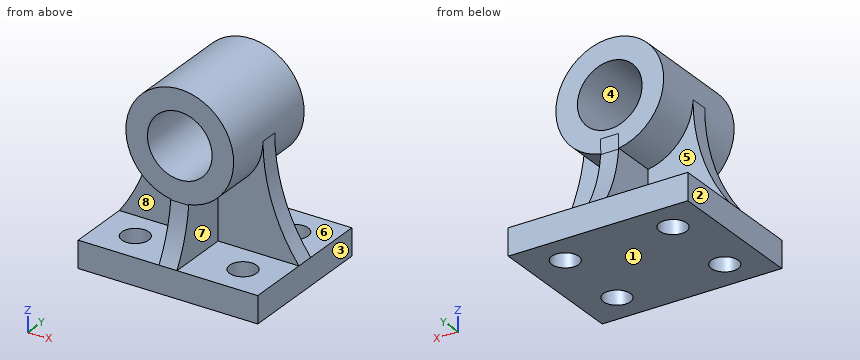
from build123d import *

# Parameters (mm, degrees)
F0_W     = 100
F0_H     = 15
F1_DEPTH = 40
F0_R     = 18
F2_DEPTH = 30
F3_DEPTH = 5
F6_DEPTH = 10
F7_R     = 7.5
F8_DEPTH = 15


with BuildPart() as f1:
    # F0 (on Front) → F1 (new body, symmetric)
    with BuildSketch(Plane.XZ):
        with Locations((50, 7.5)):
            Rectangle(F0_W, F0_H)
    extrude(amount=F1_DEPTH, both=True)



with BuildPart() as f2:
    # F0 (on Front) → F2 (new body, symmetric)
    with BuildSketch(Plane.XZ):
        with BuildLine():
            ThreePointArc((80, 75), (50, 105), (20, 75))
            ThreePointArc((20, 75), (50, 45), (80, 75))
        make_face()
        with Locations((50, 75)):
            Circle(F0_R, mode=Mode.SUBTRACT)
    extrude(amount=F2_DEPTH, both=True)


with BuildPart() as f1_1:
    add(f1.part)

    add(f2.part)  # F3 merges F2
    # F0 (on Front) → F3 (join, symmetric)
    with BuildSketch(Plane.XZ):
        with BuildLine():
            ThreePointArc((20, 75), (14.86833, 43.377223), (0, 15))
            Line((0, 15), (100, 15))
            ThreePointArc((100, 15), (85.13167, 43.377223), (80, 75))
            ThreePointArc((80, 75), (50, 45), (20, 75))
        make_face()
    extrude(amount=F3_DEPTH, both=True)

    # F5 (on offset) → F6 (join)
    with BuildSketch(Plane.YZ.offset(45)):
        with BuildLine():
            ThreePointArc((40, 15), (33.400891, 29.466964), (30, 45))
            Line((30, 45), (30.077839, 53.216796))
            Line((30.077839, 53.216796), (-30, 53.216796))
            Line((-30, 53.216796), (-30, 45))
            ThreePointArc((-30, 45), (-33.400891, 29.466964), (-40, 15))
            Line((-40, 15), (-5, 15))
            Line((-5, 15), (5, 15))
            Line((5, 15), (40, 15))
        make_face()
    extrude(amount=F6_DEPTH)

    # F7 (on face) → F8 (cut, through all)
    with BuildSketch(Plane(origin=(0, 0, 0), x_dir=(1, 0, 0), z_dir=(0, 0, -1))):
        with Locations((80, -22)):
            Circle(F7_R)
        with Locations((20, -22)):
            Circle(F7_R)
        with Locations((80, 22)):
            Circle(F7_R)
        with Locations((20, 22)):
            Circle(F7_R)
    extrude(amount=-F8_DEPTH, mode=Mode.SUBTRACT)


solid = f1_1.part
Work out the finished part from the listing and answer in its coordinate system (mm). Face numbers are marked on the shaded views. A direction names the side the tool comes from. Coordinates: 2 decimals unless noted, no trailing zeros. Loops run counter-clockwise (first coordinate to the right, second up) from the corner with the lowest first, then second, coordinate; pieces in that order, holes last. Notation, with made-up numbers: M -6,8 L 14,8 A10 ccw 14,27 Z; hole C -18.75,83.25 d5. An arc over 180 degrees is marked long. Answer in a Markdown table with one row per item. Add a question column.
1. Find section D-D, the plane z = 87. Write down the section's boundary in (x, y).
2. Find section B-B, the plane x = 50. Write down the section's boundary in (y, z).
3. Flat-ended cylindrical pins translate along their axes: P1, Ø22.5, axis at x = 27.5, z = 59, coming from the -Y side; P2, Ø3, axis at y = -6, z = 56.5, coming from the +X side; P3, Ø9, axis at x = 80, y = -22, coming from the +Z side. Find the tip coordinate at first contact, or state that the pin passes through.
4. A tool of negligible diameter and unlimited length cuts with its end or side. For the marked faces 5, 6, 7 and 8, from which of +Z, -Z, +X, -X, +Y, -Y can it reach the whole face along a straight path? Write none if from no direction.
5. The mould has two halves that part along X. Classify the marked faces 1, 2, 3 and 4: pulls with the +X half, pulls with the -X half, needs draft (parallel to the pull), parting line crosses it, or undercut.
6. Find section A-A, the plane y = 22. Write down the section's boundary in (x, z), then the cut area to 3 significant figures.
7. Find section C-C, the plane y = -6.5. Write down the section's boundary in (x, z).
8. Consider L1, parallel to X at y = -22, z = 6; L2, parallel to Y at x = 20, z = 11; L3, parallel to Z at x = 56.5, y = -22.5. Determine where each line is inside the solid, lowest interval first.
Reported:
| question | item | result |
|---|---|---|
| 1 | outline | M 22.5,-30 L 36.58,-30 L 36.58,30 L 22.5,30 Z; M 63.42,-30 L 77.5,-30 L 77.5,30 L 63.42,30 Z |
| 2 | outline | M -40,0 L 40,0 L 40,15 A75 cw 30,45 L 30.08,53.22 L 30,53.22 L 30,57 L -30,57 L -30,45 A75 cw -40,15 Z; M -30,93 L 30,93 L 30,105 L -30,105 Z |
| 3 | P1 | stops at y = -30 |
| 3 | P2 | stops at x = 81.94 |
| 3 | P3 | stops at z = 90.8 |
| 4 | face 5 | -X, +Y |
| 4 | face 6 | +X, +Y |
| 4 | face 7 | +X, -Y |
| 4 | face 8 | -X, -Y |
| 5 | face 1 | needs draft |
| 5 | face 2 | pulls with the -X half |
| 5 | face 3 | pulls with the +X half |
| 5 | face 4 | undercut |
| 6 | outline | M 0,0 L 12.5,0 L 12.5,15 L 0,15 Z; M 27.5,0 L 72.5,0 L 72.5,15 L 55,15 L 55,45.42 A30 ccw long 45,45.42 L 45,15 L 27.5,15 Z; M 87.5,0 L 100,0 L 100,15 L 87.5,15 Z; hole C 50,75 d36 |
| 6 | area | 3,160 mm^2 |
| 7 | outline | M 0,0 L 100,0 L 100,15 L 55,15 L 55,45.42 A30 ccw long 45,45.42 L 45,15 L 0,15 Z; hole C 50,75 d36 |
| 8 | L1 | x = 0 to 12.5, 27.5 to 72.5, 87.5 to 100 |
| 8 | L2 | y = -40 to -29.5, -14.5 to 14.5, 29.5 to 40 |
| 8 | L3 | z = 0 to 15, 45.71 to 58.21, 91.79 to 104.29 |
